Geometry: final body of the model. Coordinates: model frame, mm. Give positions to 0.01 mm unless a question says otherwise; leave off trailing zeros. Write each loop counter-clockwise with the first axis right and the second up, starting at its lowest first coordinate (ties: lowest second). Pieces come first, ordered by that corner, then holes. Notation, with made-up numbers: M -33,-6.75 L -16,-6.75 A34 ccw -16,25.25 Z; hole C 24,31.25 d8. An arc over 180 degrees is marked long. Use a Markdown table: item, result. Add a question column.
1) Section A-A on x = 6.5. Return the cut outline in (y, z), then the cut area to 3 significant figures.
2) Draft query along Z for faces 1 (the cylindrical face through (-1.24, -6.555, 9.444)), 2 (the flat face through (5, 0, 9)), 3 (the cylindrical face through (-1.653, -6.652, 12.592)). Return one class per face: +Z half, -Z half, draft (parallel to the pull), parting line (faces both ways), or undercut.
3) Pin query (flat end, axial travel): pin 1 (4 mm diameter, centred on y = -8.5, z = 1.5, fed in from -X); pin 2 (1.5 mm diameter, centred on y = -11.5, z = 6.5, fed in from -X); pin 3 (5 mm diameter, centred on y = -11, z = -7.5, fed in from +X); pin 4 (6 mm diameter, centred on y = -10, z = -9.5, fed in from +X). Return the tip coordinate at first contact, or that it passes through.
4) Section C-C on y = -5.75. Return the cut outline in (x, z) (3 decimals), then the cut area to 3 significant figures.
5) Line query: line 1 (Z direction, x = 0, y = -5.25) (3 decimals); line 2 (X direction, y = -9.5, z = 5.5). Output: solid intervals per line, ascending.
6) Section B-B on z = 2.5. Return the cut outline in (x, y).
7) Section D-D on x = -10.25. Return the cut outline in (y, z), then the cut area to 3 significant figures.
```python
from build123d import *

# Parameters (mm, degrees)
F0_R     = 12.7
F0_R_2   = 9.525
F1_DEPTH = 50.8
F3_DEPTH = 25.4
F4_DEPTH = 25.4


# Not quite as in the source:
# - a feature names something its author has since deleted; it is built from what else it names


with BuildPart() as f1:
    # F0 (on Front) → F1 (new body)
    with BuildSketch(Plane.XZ):
        Circle(F0_R)
        Circle(F0_R_2, mode=Mode.SUBTRACT)
    extrude(amount=F1_DEPTH)

    # F2 (on Right) → F3 (cut)
    with BuildSketch(Plane.YZ):
        Polygon((-36.6640808118, -22.974707012), (-38.1, 0), (-41.275, 50.8), (-42.5002469476, 70.4039511617), (-59.3533739448, 70.4039511617), (-59.3533739448, -22.974707012), align=None)
        Polygon((-38.1, 0), (-12.7, 0), (-15.875, 50.8), (-41.275, 50.8), align=None)
        Polygon((-11.2640808118, -22.974707012), (-12.7, 0), (-38.1, 0), (-36.6640808118, -22.974707012), align=None)
    extrude(amount=-F3_DEPTH, mode=Mode.SUBTRACT)

    # F2 (on Right) → F4 (cut)
    with BuildSketch(Plane.YZ):
        Polygon((-36.6640808118, -22.974707012), (-38.1, 0), (-41.275, 50.8), (-42.5002469476, 70.4039511617), (-59.3533739448, 70.4039511617), (-59.3533739448, -22.974707012), align=None)
        Polygon((-38.1, 0), (-12.7, 0), (-15.875, 50.8), (-41.275, 50.8), align=None)
        Polygon((-11.2640808118, -22.974707012), (-12.7, 0), (-38.1, 0), (-36.6640808118, -22.974707012), align=None)
    extrude(amount=F4_DEPTH, mode=Mode.SUBTRACT)


solid = f1.part
```
Found:
| question | item | result |
|---|---|---|
| 1 | outline | M -13.38,10.91 L -13.14,6.96 L 0,6.96 L 0,10.91 Z; M -12.26,-6.96 L -12.02,-10.91 L 0,-10.91 L 0,-6.96 Z |
| 1 | area | 100 mm² |
| 2 | face 1 | undercut |
| 2 | face 2 | draft |
| 2 | face 3 | parting line |
| 3 | pin 1 | x = -12.7 |
| 3 | pin 2 | x = -11.32 |
| 3 | pin 3 | x = 11.67 |
| 3 | pin 4 | x = 10.91 |
| 4 | outline | C 0,0 d25.4; hole C 0,0 d19.05 |
| 4 | area | 222 mm² |
| 5 | line 1 | -12.7 to -9.525, 9.525 to 12.7 |
| 5 | line 2 | -11.45 to -7.78, 7.78 to 11.45 |
| 6 | outline | M -12.45,-12.86 L -9.19,-12.86 L -9.19,0 L -12.45,0 Z; M 9.19,-12.86 L 12.45,-12.86 L 12.45,0 L 9.19,0 Z |
| 7 | outline | M -13.17,7.5 L -12.23,-7.5 L 0,-7.5 L 0,7.5 Z |
| 7 | area | 190 mm² |
